CAD build for the part. Positions are in the model's coordinates, mm. Face numbers are marked on the shaded views. A direction names the side the tool comes from. Give positions to 0.01 mm unless a question says otherwise; leave off trailing zeros. Loops run counter-clockwise (first coordinate to the right, second up) from the corner with the lowest first, then second, coordinate; pieces in that order, holes last. Notation, with made-up numbers: (64, 83.5) - (95, 83.5) arc R19 cw to (95, 105.5) - close; hole circle Ø10 at (61.5, 18). An arc over 180 degrees is marked (long way). Return JSON: item names as keys, results as strings.
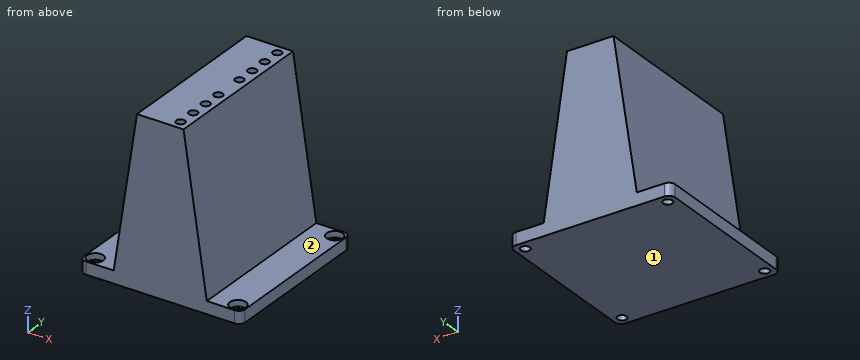
from build123d import *

# Parameters (mm, degrees)
SKETCH1_W           = 52
SKETCH1_H           = 52
BOSS_EXTRUDE1_DEPTH = 4
BOSS_EXTRUDE2_DEPTH = 52
SKETCH5_R           = 1.4
CUT_EXTRUDE4_DEPTH  = 6
SKETCH6_R           = 1.5
CUT_EXTRUDE5_DEPTH  = 6
SKETCH7_R           = 2.6
CUT_EXTRUDE6_DEPTH  = 2
FILLET1_R           = 2


with BuildPart() as part:
    # Sketch1 → Boss-Extrude1 (new body)
    with BuildSketch(Plane.XY):
        with Locations((26, 26)):
            Rectangle(SKETCH1_W, SKETCH1_H)
    extrude(amount=-BOSS_EXTRUDE1_DEPTH)

    # Sketch4 → Boss-Extrude2 (add)
    with BuildSketch(Plane(origin=(0, 52, 0), x_dir=(1, 0, 0), z_dir=(0, 1, 0))):
        Polygon((11, 0), (41, 0), (33.5, -50), (18.5, -50), align=None)
    extrude(amount=-BOSS_EXTRUDE2_DEPTH)

    # Sketch5 → Cut-Extrude4 (cut)
    with BuildSketch(Plane.XY.offset(50)):
        with Locations((30.5, 9)):
            Circle(SKETCH5_R)
        with Locations(Location((30.5, 3, 0), (0, 0, 180))):
            Circle(SKETCH5_R)
        with Locations(Location((30.5, 15, 0), (0, 0, 180))):
            Circle(SKETCH5_R)
        with Locations(Location((30.5, 21, 0), (0, 0, 180))):
            Circle(SKETCH5_R)
        with Locations((30.5, 31)):
            Circle(SKETCH5_R)
        with Locations((30.5, 37)):
            Circle(SKETCH5_R)
        with Locations((30.5, 43)):
            Circle(SKETCH5_R)
        with Locations((30.5, 49)):
            Circle(SKETCH5_R)
    extrude(amount=-CUT_EXTRUDE4_DEPTH, mode=Mode.SUBTRACT)

    # Sketch6 → Cut-Extrude5 (cut)
    with BuildSketch(Plane.XY):
        with Locations((48.980970389, 48.980970389)):
            Circle(SKETCH6_R)
        with Locations((48.980970389, 3.019029611)):
            Circle(SKETCH6_R)
        with Locations((3.019029611, 3.019029611)):
            Circle(SKETCH6_R)
        with Locations((3.019029611, 48.980970389)):
            Circle(SKETCH6_R)
    extrude(amount=-CUT_EXTRUDE5_DEPTH, mode=Mode.SUBTRACT)

    # Sketch7 → Cut-Extrude6 (cut)
    with BuildSketch(Plane.XY):
        with Locations((48.980970389, 48.980970389)):
            Circle(SKETCH7_R)
        with Locations((3.019029611, 48.980970389)):
            Circle(SKETCH7_R)
        with Locations((3.019029611, 3.019029611)):
            Circle(SKETCH7_R)
        with Locations((48.980970389, 3.019029611)):
            Circle(SKETCH7_R)
    extrude(amount=-CUT_EXTRUDE6_DEPTH, mode=Mode.SUBTRACT)

    # Fillet1
    fillet1_edges = [part.edges().sort_by_distance(p)[0] for p in [
        (0, 0, -2),
        (0, 52, -2),
        (52, 52, -2),
        (52, 0, -2),
    ]]
    fillet(fillet1_edges, radius=FILLET1_R)


solid = part.part
1. Drop flat-ended pins along their axis: P1, Ø3, axis at x = 30.5, y = 37, coming from the +Z side; P2, Ø3, axis at y = 19, z = 12, coming from the -X side (3 decimals); P3, Ø4, axis at x = 48, y = 2, coming from the +Z side; P4, Ø4, axis at x = 3.02, y = 3.02, coming from the +Z side. Give the stop position or say it passes through.
Values follow:
{"P1": "stops at z = 50", "P2": "stops at x = 12.575", "P3": "stops at z = 0", "P4": "stops at z = -2"}
2. Cut at B-B, the plane z = 22. Write the cut outline in (x, y), plus the area to 3 significant figures.
Values follow:
{"outline": "(14.3, 0) - (37.7, 0) - (37.7, 52) - (14.3, 52) - close", "area": "1,220 mm²"}
3. Which spindle directions (+Z, -Z, +X, -X, +Y, -Y) get a long thin tool onto all of the face, cutting with end or side? Do the marked faces 1 and 2. Say none if no direction does.
Values follow:
{"face 1": "-Z, +X, -X, +Y, -Y", "face 2": "+Z, +X, +Y, -Y"}
4. Drill centre lines: probe 1 along Z at (x, y) = (5, 23); probe 2 along X at (y, z) = (3, 46); probe 3 along X at (y, z) = (21, 48.6). Where is each one in solid material? Low to high.
Values follow:
{"probe 1": "z = -4 to 0", "probe 2": "x = 17.9 to 29.1, 31.9 to 34.1", "probe 3": "x = 18.29 to 29.1, 31.9 to 33.71"}
5. Cut at A-A, the plane y = 31. Write the cut outline in (x, z), plus the area to 3 significant figures.
Values follow:
{"outline": "(0, -4) - (52, -4) - (52, 0) - (41, 0) - (33.5, 50) - (31.9, 50) - (31.9, 44) - (29.1, 44) - (29.1, 50) - (18.5, 50) - (11, 0) - (0, 0) - close", "area": "1,320 mm²"}
6. Cut at C-C, the plane x = 9.5. Write the cut outline in (y, z).
Values follow:
{"outline": "(0, -4) - (52, -4) - (52, 0) - (0, 0) - close"}
